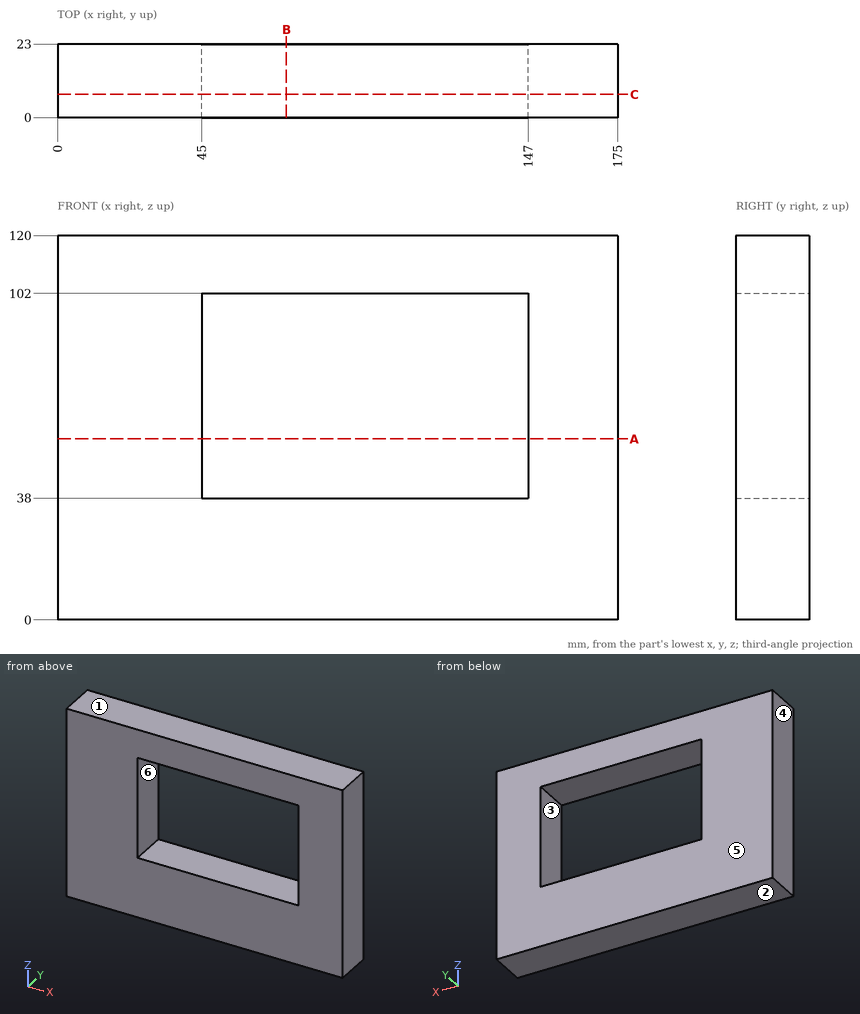
Here's the drawing with two shaded views (mm, measured from the low corner). I have some questions. A direction names the side the tool comes from. Give positions to 0.01 mm unless a question says otherwise; leave off trailing zeros. Write each loop counter-clockwise with the first axis right and the second up, starting at its lowest first coordinate (ties: lowest second). Pieces come first, ordered by that corner, then holes. Notation, with made-up numbers: (78.5, 67) -> (89.5, 67) arc R23 ccw to (89.5, 95) -> close; hole circle Ø8 at (9.25, 74). An arc over 180 degrees is marked (long way). Use one line per item in the form item = value.
1) Suppose I cut it at A-A (z = 56.5). Please give me the cut outline in (x, y), and give its area (3 significant figures).
Verdict:
outline = (0, 0) -> (45, 0) -> (45, 23) -> (0, 23) -> close; (147, 0) -> (175, 0) -> (175, 23) -> (147, 23) -> close
area = 1,680 mm2
2) Suppose I cut it at B-B (x = 71.5). Please give me the cut outline in (y, z).
Verdict:
outline = (0, 0) -> (23, 0) -> (23, 38) -> (0, 38) -> close; (0, 102) -> (23, 102) -> (23, 120) -> (0, 120) -> close
3) Suppose I cut it at C-C (y = 7.25). Please give me the cut outline in (x, z), and give its area (3 significant figures).
Verdict:
outline = (0, 0) -> (175, 0) -> (175, 120) -> (0, 120) -> close; hole (45, 38) -> (147, 38) -> (147, 102) -> (45, 102) -> close
area = 14,500 mm2
4) We'd pull the mould along Z, two halves only. Please class the marked faces 1, 2, 3 and 4: +Z half, -Z half, draft (parallel to the pull), parting line (faces both ways), or undercut.
Verdict:
face_1 = +Z half
face_2 = -Z half
face_3 = undercut
face_4 = draft
5) On a 3-axis mill with a long thin cutter (end or side, diameter ignored), from which of +Z, -Z, +X, -X, +Y, -Y can I reach the whole of each face in a straight line? I mean the marked faces 5 and 6. Say none if no direction works.
Verdict:
face_5 = +Z, -Z, +X, -X, +Y
face_6 = +Y, -Y
6) If I drill on L1, parallel to Z at x = 65, y = 12; L2, parallel to X at y = 13, z = 80, over which ranges is the centre line in solid material (lowest first)? Write a range as [from, to].
Verdict:
L1 = [0, 38], [102, 120]
L2 = [0, 45], [147, 175]
